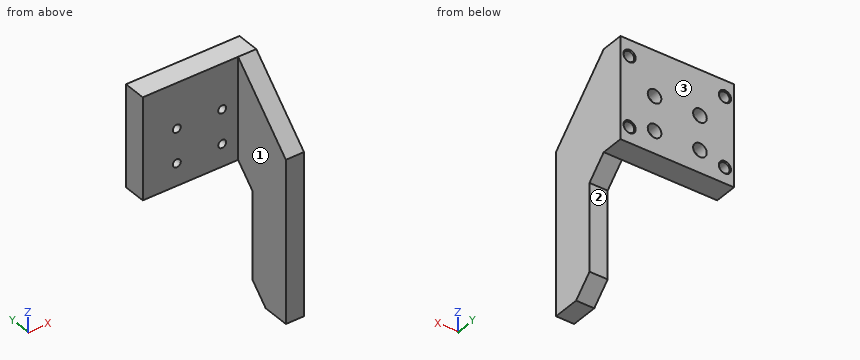
```python
from build123d import *

# Parameters (mm, degrees)
SKETCH1_W               = 50
SKETCH1_H               = 34.7
BOSS_EXTRUDE1_DEPTH     = 10
CUT_EXTRUDE1_REACH      = 34.032
SKETCH2_R               = 1.75
SKETCH3_R               = 3
CUT_EXTRUDE2_DEPTH      = 5
SKETCH6_W               = 50
SKETCH6_H               = 10
BOSS_EXTRUDE3_DEPTH     = 10
BOSS_EXTRUDE4_DEPTH     = 8
CHAMFER1_SIZE           = 8
SKETCH10_R              = 2.3
CUT_EXTRUDE3_DEPTH      = 4.8
MIRROR2_COPY_1_SKETCH_R = 2.3
MIRROR2_COPY_1_DEPTH    = 4.8
CHAMFER2_SIZE           = 0.4


with BuildPart() as part:
    # Sketch1 → Boss-Extrude1 (new body)
    with BuildSketch(Plane(origin=(0, 0, 0), x_dir=(1, 0, 0), z_dir=(0, 1, 0))):
        Rectangle(SKETCH1_W, SKETCH1_H)
    extrude(amount=BOSS_EXTRUDE1_DEPTH)

    # Sketch2 → Cut-Extrude1 (cut, up to next)
    with BuildSketch(Plane(origin=(0, 10, 0), x_dir=(1, 0, 0), z_dir=(0, 1, 0)), mode=Mode.PRIVATE) as cut_extrude1_sk1:
        with Locations(Location((-10, 7.5, 0), (0, 0, 270))):
            Circle(SKETCH2_R)
    cut_extrude1_tool1 = extrude(cut_extrude1_sk1.sketch, amount=-CUT_EXTRUDE1_REACH, mode=Mode.PRIVATE) & part.part
    # Sketch2 → Cut-Extrude1 (cut, up to next)
    with BuildSketch(Plane(origin=(0, 10, 0), x_dir=(1, 0, 0), z_dir=(0, 1, 0)), mode=Mode.PRIVATE) as cut_extrude1_sk2:
        with Locations(Location((10, 7.5, 0), (0, 0, 270))):
            Circle(SKETCH2_R)
    cut_extrude1_tool2 = extrude(cut_extrude1_sk2.sketch, amount=-CUT_EXTRUDE1_REACH, mode=Mode.PRIVATE) & part.part
    # Sketch2 → Cut-Extrude1 (cut, up to next)
    with BuildSketch(Plane(origin=(0, 10, 0), x_dir=(1, 0, 0), z_dir=(0, 1, 0)), mode=Mode.PRIVATE) as cut_extrude1_sk3:
        with Locations(Location((10, -7.5, 0), (0, 0, 270))):
            Circle(SKETCH2_R)
    cut_extrude1_tool3 = extrude(cut_extrude1_sk3.sketch, amount=-CUT_EXTRUDE1_REACH, mode=Mode.PRIVATE) & part.part
    # Sketch2 → Cut-Extrude1 (cut, up to next)
    with BuildSketch(Plane(origin=(0, 10, 0), x_dir=(1, 0, 0), z_dir=(0, 1, 0)), mode=Mode.PRIVATE) as cut_extrude1_sk4:
        with Locations(Location((-10, -7.5, 0), (0, 0, 270))):
            Circle(SKETCH2_R)
    cut_extrude1_tool4 = extrude(cut_extrude1_sk4.sketch, amount=-CUT_EXTRUDE1_REACH, mode=Mode.PRIVATE) & part.part
    add(cut_extrude1_tool1.solids().sort_by_distance((-10, 10, -7.5))[0], mode=Mode.SUBTRACT)
    add(cut_extrude1_tool2.solids().sort_by_distance((10, 10, -7.5))[0], mode=Mode.SUBTRACT)
    add(cut_extrude1_tool3.solids().sort_by_distance((10, 10, 7.5))[0], mode=Mode.SUBTRACT)
    add(cut_extrude1_tool4.solids().sort_by_distance((-10, 10, 7.5))[0], mode=Mode.SUBTRACT)

    # Sketch3 → Cut-Extrude2 (cut)
    with BuildSketch(Plane(origin=(0, 10, 0), x_dir=(1, 0, 0), z_dir=(0, 1, 0))):
        with Locations(Location((-10, 7.5, 0), (0, 0, 270))):
            Circle(SKETCH3_R)
        with Locations(Location((10, 7.5, 0), (0, 0, 270))):
            Circle(SKETCH3_R)
        with Locations(Location((10, -7.5, 0), (0, 0, 270))):
            Circle(SKETCH3_R)
        with Locations(Location((-10, -7.5, 0), (0, 0, 270))):
            Circle(SKETCH3_R)
    extrude(amount=-CUT_EXTRUDE2_DEPTH, mode=Mode.SUBTRACT)

    # Sketch6 → Boss-Extrude3 (add)
    with BuildSketch(Plane.XZ):
        with Locations((0, 22.35)):
            Rectangle(SKETCH6_W, SKETCH6_H)
    extrude(amount=-BOSS_EXTRUDE3_DEPTH)

    # Sketch8 → Boss-Extrude4 (add)
    with BuildSketch(Plane(origin=(25, 0, 0), x_dir=(0, 0, -1), z_dir=(1, 0, 0))):
        Polygon((-27.35, 0), (17.35, 0), (25.85, -8.5), (72.35, -8.5), (72.35, -28.5), (1.15, -28.5), align=None)
    extrude(amount=-BOSS_EXTRUDE4_DEPTH)

    # Chamfer1
    chamfer1_edges = [part.edges().sort_by_distance(p)[0] for p in [
        (21, -8.5, -72.35),
    ]]
    chamfer(chamfer1_edges, length=CHAMFER1_SIZE)

    # Sketch10 → Cut-Extrude3 (cut)
    with BuildSketch(Plane(origin=(0, 10, 0), x_dir=(1, 0, 0), z_dir=(0, 1, 0))):
        with Locations(Location((21, 10.35, 0), (0, 0, 270))):
            Circle(SKETCH10_R)
    cut_extrude3 = extrude(amount=-CUT_EXTRUDE3_DEPTH, mode=Mode.SUBTRACT)

    # Mirror1: Cut-Extrude3 across plane
    add(cut_extrude3.mirror(Plane(origin=(0, 0, 5), x_dir=(1, 0, 0), z_dir=(0, 0, -1))), mode=Mode.SUBTRACT)

    # Mirror2: Cut-Extrude3 across plane
    add(cut_extrude3.mirror(Plane.ZY), mode=Mode.SUBTRACT)

    # Mirror2 copy 1 sketch → Mirror2 copy 1 (cut)
    with BuildSketch(Plane(origin=(0, 10, 10), x_dir=(-1, 0, 0), z_dir=(0, 1, 0))):
        with Locations(Location((21, 10.35, 0), (0, 0, 270))):
            Circle(MIRROR2_COPY_1_SKETCH_R)
    extrude(amount=-MIRROR2_COPY_1_DEPTH, mode=Mode.SUBTRACT)

    # Chamfer2
    chamfer2_edges = [part.edges().sort_by_distance(p)[0] for p in [
        (-21, 10, -12.65),
        (-21, 10, 22.65),
        (21, 10, -12.65),
        (21, 10, 22.65),
    ]]
    chamfer(chamfer2_edges, length=CHAMFER2_SIZE)


solid = part.part
```
Input: part model. Units: mm. Frame: model coordinates. Face numbers are marked on the shaded views. A direction names the side the tool comes from. Round coordinates to 2 decimals unless told otherwise and drop trailing zeros. Write each loop counter-clockwise with the first axis right and the second up, starting at its lowest first coordinate (ties: lowest second). Pieces come first, ordered by that corner, then holes. Notation, with made-up numbers: (-15, -26.5) -> (5, -26.5) arc R34 cw to (5, 6.5) -> close; hole circle Ø11 at (89.25, 56). An arc over 180 degrees is marked (long way). Answer as CSV lines item,"result".
1. Section B-B (x = -10). Return the cut outline in (y, z).
Geometry says:
outline,"(0, -17.35) -> (10, -17.35) -> (10, -10.5) -> (5, -10.5) -> (5, -9.25) -> (0, -9.25) -> close; (0, -5.75) -> (5, -5.75) -> (5, -4.5) -> (10, -4.5) -> (10, 4.5) -> (5, 4.5) -> (5, 5.75) -> (0, 5.75) -> close; (0, 9.25) -> (5, 9.25) -> (5, 10.5) -> (10, 10.5) -> (10, 27.35) -> (0, 27.35) -> close"
2. Section C-C (y = 1.5). Return the cut outline in (x, z).
Geometry says:
outline,"(-25, -17.35) -> (25, -17.35) -> (25, 27.35) -> (-25, 27.35) -> close; hole circle Ø3.5 at (-10, -7.5); hole circle Ø3.5 at (-10, 7.5); hole circle Ø3.5 at (10, -7.5); hole circle Ø3.5 at (10, 7.5)"
3. Reachability of the marked faces 1, 2 and 3 from +Z, -Z, +X, -X, +Y, -Y: full face, straight path, thin tool, end or side. Return the list, or none.
Geometry says:
face 1,"+Z, -Z, -X, -Y"
face 2,"-Z, +X, -X, +Y"
face 3,"+Z, -Z, +X, -X, +Y"
4. Section A-A (z = 7.5). Return the cut outline in (x, y), plus the area to 3 significant figures.
Geometry says:
outline,"(-25, 0) -> (-11.75, 0) -> (-11.75, 5) -> (-13, 5) -> (-13, 10) -> (-25, 10) -> close; (-8.25, 0) -> (8.25, 0) -> (8.25, 5) -> (7, 5) -> (7, 10) -> (-7, 10) -> (-7, 5) -> (-8.25, 5) -> close; (11.75, 0) -> (17, 0) -> (17, -19.85) -> (25, -19.85) -> (25, 10) -> (13, 10) -> (13, 5) -> (11.75, 5) -> close"
area,"564 mm^2"
5. Ray query, L1, parallel to X at y = 7.85, z = -7.5; L2, parallel to Z at x = -21, y = 7.05; L3, parallel to Y at x = 19.5, z = -37.5. Return the intervals inside material, ascending. Write a range as [from, to].
Geometry says:
L1,"x = [-25, -13], [-7, 7], [13, 25]"
L2,"z = [-17.35, -12.65], [-8.05, 18.05], [22.65, 27.35]"
L3,"y = [-28.5, -8.5]"
6. Contact query for flat-ended pins moving along their axis: P1, Ø5.5, axis at x = -21, z = 20.35, coming from the -Y side; P2, Ø9.5, axis at x = -10, z = -7.5, coming from the +Y side; P3, Ø5, axis at x = 10, z = -7.5, coming from the +Y side; P4, Ø10, axis at x = -9, y = 4.5, coming from the -Z side. Output: stop coordinate, or through.
Geometry says:
P1,"stops at y = 0"
P2,"stops at y = 10"
P3,"stops at y = 5"
P4,"stops at z = -17.35"
7. Section D-D (z = 20.35). Return the cut outline in (x, y), plus the area to 3 significant figures.
Geometry says:
outline,"(-25, 0) -> (17, 0) -> (17, -7) -> (25, -7) -> (25, 10) -> (23.7, 10) -> (23.3, 9.6) -> (23.3, 5.2) -> (18.7, 5.2) -> (18.7, 9.6) -> (18.3, 10) -> (-18.3, 10) -> (-18.7, 9.6) -> (-18.7, 5.2) -> (-23.3, 5.2) -> (-23.3, 9.6) -> (-23.7, 10) -> (-25, 10) -> close"
area,"512 mm^2"
